Autodesk Inventor part; units mm, degrees
ref_plane "YZ Plane" through (0, 0, 0) normal (1, 0, 0) x (0, 1, 0)
ref_plane "XZ Plane" through (0, 0, 0) normal (0, 1, 0) x (-1, 0, 0)
ref_plane "XY Plane" through (0, 0, 0) normal (0, 0, 1) x (1, 0, 0)
sketch "Эскиз1" plane through (0, 0, 0) normal (0, 0, 1) x (1, 0, 0)
  circle A0 centre (0, 0) radius 40
  dimension "d0" = 80
extrude "Выдавливание1" add sketch "Эскиз1" along normal blind 25
sketch "Эскиз2" plane through (0, 0, 25) normal (0, 0, 1) x (1, 0, 0)
  point P0 (0, 0)
  point P1 (-30, 0)
  point P2 (30, 0)
  dimension "d3" = 30
  dimension "d4" = 60
hole "Отверстие1" at (-30, 0, 25) at (30, 0, 25) direction (0, 0, -1) diameter 6.647 depth 16.75 tip angle 120
chamfer "Фаска1" distance 1.6 angle 45 2 edges at (-30, 3.3235, 25) (30, 3.3235, 25)
sketch "Эскиз3" plane through (0, 0, 25) normal (0, 0, 1) x (1, 0, 0)
  circle A0 centre (0, 0) radius 22
  dimension "d15" = 44
extrude "Выдавливание2" cut sketch "Эскиз3" against normal blind 9
sketch "Эскиз4" plane through (0, 0, 16) normal (0, 0, 1) x (1, 0, 0)
  circle A0 centre (0, 0) radius 16
  dimension "d18" = 32
extrude "Выдавливание3" cut sketch "Эскиз4" against normal through all
sketch "Эскиз5" plane through (0, 0, 0) normal (0, 0, -1) x (-1, 0, 0)
  circle A0 centre (0, 0) radius 24
  dimension "d21" = 48
extrude "Выдавливание4" cut sketch "Эскиз5" against normal blind 6
properties part number "Корпус"
Work out the finished part from the listing and answer in its coordinate system (mm). A direction names the side the tool comes from. Round coordinates to 2 decimals unless told otherwise and drop trailing zeros. Write each loop counter-clockwise with the first axis right and the second up, starting at its lowest first coordinate (ties: lowest second). Pieces come first, ordered by that corner, then holes. Notation, with made-up numbers: (-39.5, 66) -> (-1.5, 66) arc R7 ccw to (-1.5, 79) -> close; hole circle Ø7 at (63, 42). An arc over 180 degrees is marked (long way). Write each question's results on one line, items separated by ' | '.
Item 1: The mould has two halves that part along Y. Classify faces 1 (the face through (17.2, -17.2, 0)), 2 (the face through (-8.67, 39.05, 12.32)), 3 (the face through (29.488, -0.266, 6.664)), 4 (the face through (26.7, 0.4, 15.7)): +Y half, -Y half, draft (parallel to the pull), parting line (faces both ways), or undercut.
Result set:
face 1: draft | face 2: parting line | face 3: undercut | face 4: undercut
Item 2: Find the intervals of material crossed by line 1 along Y through (x, z) = (0, 1.8); line 2 along Y through (x, z) = (-20.5, 5.5); line 3 along Z through (x, y) = (3, 23), in increasing order. Write a range as [from, to].
Result set:
line 1: [-40, -24], [24, 40] | line 2: [-34.35, -12.48], [12.48, 34.35] | line 3: [6, 25]
Item 3: A cutting plane is placed at A-A, the plane x = -10. Determine the outline of the cut face in (y, z), plus the area to 3 significant figures.
Result set:
outline: (-38.73, 0) -> (-21.82, 0) -> (-21.82, 6) -> (-12.49, 6) -> (-12.49, 16) -> (-19.6, 16) -> (-19.6, 25) -> (-38.73, 25) -> close; (12.49, 6) -> (21.82, 6) -> (21.82, 0) -> (38.73, 0) -> (38.73, 25) -> (19.6, 25) -> (19.6, 16) -> (12.49, 16) -> close | area: 1,070 mm^2
Item 4: Which of the six approach directions +Z, -Z, +X, -X, +Y, -Y give full straight-line access (tool end or side, diameter ignored) to faces 5 (the face through (-3.47, -15.62, 11.07)), 6 (the face through (-5, -16, 6)), 7 (the face through (-33.3, 0.4, 15.7))?
Result set:
face 5: +Z, -Z | face 6: -Z | face 7: +Z
Item 5: A cutting plane is placed at B-B, the plane z = 22. Determine the outline of the cut face in (x, y), plus the area to 3 significant figures.
Result set:
outline: circle Ø80 at (0, 0); hole circle Ø6.65 at (-30, 0); hole circle Ø44 at (0, 0); hole circle Ø6.65 at (30, 0) | area: 3,440 mm^2
Item 6: A cutting plane is placed at C-C, the plane x = 18. Determine the outline of the cut face in (y, z).
Result set:
outline: (-35.72, 0) -> (-15.87, 0) -> (-15.87, 6) -> (15.87, 6) -> (15.87, 0) -> (35.72, 0) -> (35.72, 25) -> (12.65, 25) -> (12.65, 16) -> (-12.65, 16) -> (-12.65, 25) -> (-35.72, 25) -> close
Item 7: Flat-ended cylindrical pins translate along their axes: P1, Ø1, axis at x = 7.5, y = 15, coming from the +Z side; P2, Ø1, axis at x = 29, z = 8, coming from the -Y side; P3, Ø1.5, axis at x = -30, z = 20.5, coming from the +Y side. Find the tip coordinate at first contact, or state that the pin passes through.
Result set:
P1: z = 16 | P2: y = -28.07 | P3: y = 27.28
Item 8: A cutting plane is placed at D-D, the plane y = 32. Determine the outline of the cut face in (x, z).
Result set:
outline: (-24, 0) -> (24, 0) -> (24, 25) -> (-24, 25) -> close
